```python
from build123d import *

# Parameters (mm, degrees)
SKETCH1_R           = 22
BOSS_EXTRUDE1_DEPTH = 2.4
SKETCH2_R           = 11
BOSS_EXTRUDE2_DEPTH = 5
SKETCH3_R           = 3.9
BOSS_EXTRUDE3_DEPTH = 9
BOSS_EXTRUDE4_START = 20.6
SKETCH4_R           = 11
BOSS_EXTRUDE4_DEPTH = 20.6
SKETCH5_R           = 2.7
CUT_EXTRUDE1_DEPTH  = 39.691084244


with BuildPart() as part:
    # Sketch1 → Boss-Extrude1 (new body)
    with BuildSketch(Plane(origin=(0, 0, 0), x_dir=(1, 0, 0), z_dir=(0, 1, 0))):
        with Locations(Location((0, 0, 0), (0, 0, 270))):
            Circle(SKETCH1_R)
    extrude(amount=BOSS_EXTRUDE1_DEPTH)

    # Sketch2 → Boss-Extrude2 (add)
    with BuildSketch(Plane(origin=(0, 2.4, 0), x_dir=(1, 0, 0), z_dir=(0, 1, 0))):
        with Locations(Location((0, 0, 0), (0, 0, 270))):
            Circle(SKETCH2_R)
    extrude(amount=BOSS_EXTRUDE2_DEPTH)

    # Sketch3 → Boss-Extrude3 (add)
    with BuildSketch(Plane(origin=(0, 7.4, 0), x_dir=(1, 0, 0), z_dir=(0, 1, 0))):
        with Locations(Location((0, 0, 0), (0, 0, 270))):
            Circle(SKETCH3_R)
    extrude(amount=BOSS_EXTRUDE3_DEPTH)

    # Sketch4 → Boss-Extrude4 (add)
    with BuildSketch(Plane.XZ.offset(BOSS_EXTRUDE4_START)):
        with Locations(Location((0, 0, 0), (0, 0, 90))):
            Circle(SKETCH4_R)
    extrude(amount=-BOSS_EXTRUDE4_DEPTH)

    # Sketch5 → Cut-Extrude1 (cut, through all)
    with BuildSketch(Plane(origin=(0, 2.4, 0), x_dir=(1, 0, 0), z_dir=(0, 1, 0))):
        with Locations(Location((0, 17.5, 0), (0, 0, 270))):
            Circle(SKETCH5_R)
        with Locations(Location((-15.155444566, -8.75, 0), (0, 0, 270))):
            Circle(SKETCH5_R)
        with Locations(Location((15.155444566, -8.75, 0), (0, 0, 270))):
            Circle(SKETCH5_R)
    extrude(amount=-CUT_EXTRUDE1_DEPTH, mode=Mode.SUBTRACT)


solid = part.part
```
The model under review builds one solid part; all positions refer to its coordinate system, in mm. A direction names the side the tool comes from. Give positions to 0.01 mm unless a question says otherwise; leave off trailing zeros. Write each loop counter-clockwise with the first axis right and the second up, starting at its lowest first coordinate (ties: lowest second). Pieces come first, ordered by that corner, then holes. Notation, with made-up numbers: (-38.5, -23.75) -> (-34.5, -23.75) arc R19 ccw to (-34.5, -14.75) -> close; hole circle Ø9 at (2.25, 4). An arc over 180 degrees is marked (long way). Put each result on its own line as item: value.
(1) For pin 1 Ø1.5 at (x, z) = (16, -6) entering from +Y; pin 2 Ø8.5 at (x, z) = (15.16, 8.75) entering from -Y; pin 3 Ø6.5 at (x, z) = (1.5, 4.5) entering from +Y; pin 4 Ø1.5 at (y, z) = (-13, -3.5) entering from +X, all flat-tipped, find the tip position at first contact; note any pin that passes through.
Results are:
pin 1: y = 2.4
pin 2: y = 0
pin 3: y = 16.4
pin 4: x = 10.65
(2) The part is to be moulded in two halves that separate along X. For faces 1 (the cylindrical face through (0.811, 1.217, -14.925)), 2 (the flat face through (10, 2.4, 5)), 3 (the cylindrical face through (-21.477, 1.183, -4.769)), say which applies: pulls with the +X half, pulls with the -X half, needs draft (parallel to the pull), parting line crosses it, or undercut.
Results are:
face 1: undercut
face 2: needs draft
face 3: parting line crosses it
(3) We need section C-C, the plane z = -17.5. Give the boundary of the cut face in (x, y), and give its area (3 significant figures).
Results are:
outline: (-13.33, 0) -> (-2.7, 0) -> (-2.7, 2.4) -> (-13.33, 2.4) -> close; (2.7, 0) -> (13.33, 0) -> (13.33, 2.4) -> (2.7, 2.4) -> close
area: 51.0 mm²
(4) We need section A-A, the plane z = 0. Give the boundary of the cut face in (x, y), and give its area (3 significant figures).
Results are:
outline: (-22, 0) -> (-11, 0) -> (-11, -20.6) -> (11, -20.6) -> (11, 0) -> (22, 0) -> (22, 2.4) -> (11, 2.4) -> (11, 7.4) -> (3.9, 7.4) -> (3.9, 16.4) -> (-3.9, 16.4) -> (-3.9, 7.4) -> (-11, 7.4) -> (-11, 2.4) -> (-22, 2.4) -> close
area: 739 mm²
(5) Tool access review of faces 4 (the cylindrical face through (10.74, -10.44, -2.38)), 5 (the cylindrical face through (-10.74, 4.86, -2.38)), 6 (the flat face through (0, -20.6, 0)): name each direction out of +Z, -Z, +X, -X, +Y, -Y from which nothing blocks a thin tool from reaching the whole face with its end or side.
Results are:
face 4: -Y
face 5: +Y
face 6: +Z, -Z, +X, -X, -Y
(6) We need section B-B, the plane x = 0. Give the boundary of the cut face in (y, z).
Results are:
outline: (-20.6, -11) -> (0, -11) -> (0, -14.8) -> (2.4, -14.8) -> (2.4, -11) -> (7.4, -11) -> (7.4, -3.9) -> (16.4, -3.9) -> (16.4, 3.9) -> (7.4, 3.9) -> (7.4, 11) -> (2.4, 11) -> (2.4, 22) -> (0, 22) -> (0, 11) -> (-20.6, 11) -> close; (0, -22) -> (2.4, -22) -> (2.4, -20.2) -> (0, -20.2) -> close
(7) We need section D-D, the plane z = 8.75. Give the boundary of the cut face in (x, y), and give its area (3 significant figures).
Results are:
outline: (-20.19, 0) -> (-17.86, 0) -> (-17.86, 2.4) -> (-20.19, 2.4) -> close; (-12.46, 0) -> (-6.67, 0) -> (-6.67, -20.6) -> (6.67, -20.6) -> (6.67, 0) -> (12.46, 0) -> (12.46, 2.4) -> (6.67, 2.4) -> (6.67, 7.4) -> (-6.67, 7.4) -> (-6.67, 2.4) -> (-12.46, 2.4) -> close; (17.86, 0) -> (20.19, 0) -> (20.19, 2.4) -> (17.86, 2.4) -> close
area: 412 mm²
(8) To check wall thickness, follow probe 1 along X at (y, z) = (0.7, 8.75); probe 2 along Y at (x, z) = (-7, -15); probe 3 along Z at (x, y) = (15.5, 2). State the ranges of each line that lie inside material, in increasing order. Write a range as from..to.
Results are:
probe 1: -20.19..-17.86, -12.46..12.46, 17.86..20.19
probe 2: 0..2.4
probe 3: -15.61..6.07, 11.43..15.61
